Verification items for the finished model (mm, model axes). Face numbers are marked on the shaded views. A direction names the side the tool comes from. Coordinates: 2 decimals unless noted, no trailing zeros. Order: outer loops, then holes, each group sorted by start corner. A loop starts at its lowest first (then second) coordinate and runs counter-clockwise, first axis right, second up. Notation, with made-up numbers: (15, 1) - (42, 1) arc R35 ccw to (42, 36) - close; hole circle Ø10 at (61.5, 19). An arc over 180 degrees is marked (long way). Answer as CSV lines item,"result". Start each with the question number.
1. Mould release check, pull along X, two halves, no side actions. Record for the marked faces 1, 2 and 3: pulls with the +X half, pulls with the -X half, needs draft (parallel to the pull), parting line crosses it, or undercut.
2. Material ranges on L1, parallel to X at y = -29, z = 68; L2, parallel to Z at x = 149.5, y = -46.5, recorded low to high. Write a range as [from, to].
3. Go/stop test with a flat-tipped pin: pin 1 (10 mm diameter, centred on x = 179, y = 6, fed in from -Z). Record where the tip stops, or that it passes through.
4. Section check A-A (z = 56). Record the cut outline in (x, y), and give its area (3 significant figures).
5. Set-up check for the marked faces 4 and 5: record each of +Z, -Z, +X, -X, +Y, -Y from which the full face is reachable in a straight line by a thin tool's end or side.
6. Section check C-C (x = 936). Record the cut outline in (y, z), and give its area (3 significant figures).
7. Section check B-B (y = -63.5). Record the cut outline in (x, z), and give its area (3 significant figures).
from build123d import *

# Parameters (mm, degrees)
SKETCH1_W           = 76.2
SKETCH1_H           = 152.4
BOSS_EXTRUDE1_DEPTH = 1219.2
SKETCH2_W           = 152.4
SKETCH2_H           = 152.4
BOSS_EXTRUDE2_DEPTH = 12.7
SKETCH3_W           = 152.4
SKETCH3_H           = 152.4
BOSS_EXTRUDE3_DEPTH = 12.7


with BuildPart() as part:
    # Sketch1 → Boss-Extrude1 (new body)
    with BuildSketch(Plane(origin=(0, 0, 0), x_dir=(0, 0, -1), z_dir=(1, 0, 0))):
        Rectangle(SKETCH1_W, SKETCH1_H)
    extrude(amount=BOSS_EXTRUDE1_DEPTH)

    # Sketch2 → Boss-Extrude2 (add)
    with BuildSketch(Plane(origin=(1219.2, 0, 0), x_dir=(0, 0, -1), z_dir=(1, 0, 0))):
        Rectangle(SKETCH2_W, SKETCH2_H)
    extrude(amount=-BOSS_EXTRUDE2_DEPTH)

    # Sketch3 → Boss-Extrude3 (add)
    with BuildSketch(Plane.ZY):
        Rectangle(SKETCH3_W, SKETCH3_H)
    extrude(amount=-BOSS_EXTRUDE3_DEPTH)


solid = part.part
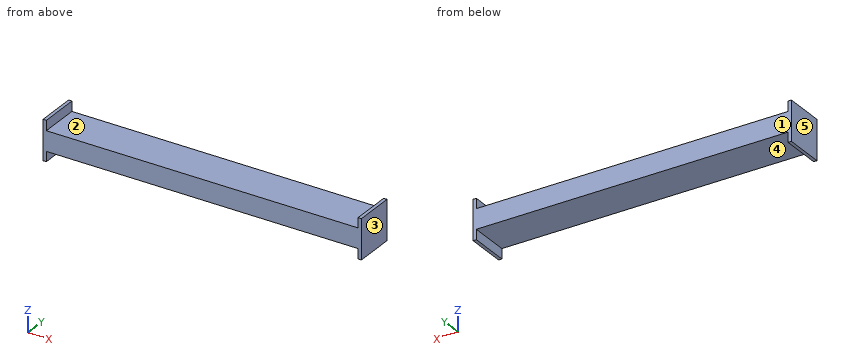
Evaluation:
1,face 1,"needs draft"
1,face 2,"undercut"
1,face 3,"pulls with the +X half"
2,L1,"x = [0, 12.7], [1206.5, 1219.2]"
2,L2,"z = [-38.1, 38.1]"
3,pin 1,"stops at z = -38.1"
4,outline,"(0, -76.2) - (12.7, -76.2) - (12.7, 76.2) - (0, 76.2) - close; (1206.5, -76.2) - (1219.2, -76.2) - (1219.2, 76.2) - (1206.5, 76.2) - close"
4,area,"3,870 mm²"
5,face 4,"-Z, +Y, -Y"
5,face 5,"+Z, -Z, -X, +Y, -Y"
6,outline,"(-76.2, -38.1) - (76.2, -38.1) - (76.2, 38.1) - (-76.2, 38.1) - close"
6,area,"11,600 mm²"
7,outline,"(0, -76.2) - (12.7, -76.2) - (12.7, -38.1) - (1206.5, -38.1) - (1206.5, -76.2) - (1219.2, -76.2) - (1219.2, 76.2) - (1206.5, 76.2) - (1206.5, 38.1) - (12.7, 38.1) - (12.7, 76.2) - (0, 76.2) - close"
7,area,"94,800 mm²"
